```python
from build123d import *

# Parameters (mm, degrees)
BOSS_EXTRUDE1_DEPTH = 49.53
CUT_EXTRUDE1_DEPTH  = 44.45
SKETCH3_R           = 4.7625
CUT_EXTRUDE2_DEPTH  = 44.45


with BuildPart() as part:
    # Sketch1 → Boss-Extrude1 (new body)
    with BuildSketch(Plane(origin=(0, 0, 0), x_dir=(1, 0, 0), z_dir=(0, 1, 0))):
        Polygon((-12.7, -12.7), (-10.795, -12.7), (-10.795, -1.905), (10.795, -1.905), (10.795, -12.7), (12.7, -12.7), (12.7, 0), (-12.7, 0), align=None)
    extrude(amount=BOSS_EXTRUDE1_DEPTH)

    # Sketch2 → Cut-Extrude1 (cut)
    with BuildSketch(Plane(origin=(12.7, 0, 0), x_dir=(0, 0, -1), z_dir=(1, 0, 0))):
        with BuildLine():
            Line((-12.7, 0), (-8.821918242, 37.623946857))
            ThreePointArc((-8.821918242, 37.623946857), (-4.512325964, 46.11357553), (4.374429599, 49.53))
            Line((4.374429599, 49.53), (-12.7, 49.53))
            Line((-12.7, 49.53), (-12.7, 0))
        make_face()
    extrude(amount=-CUT_EXTRUDE1_DEPTH, mode=Mode.SUBTRACT)

    # Sketch3 → Cut-Extrude2 (cut)
    with BuildSketch(Plane(origin=(0, 0, 0), x_dir=(-1, 0, 0), z_dir=(0, 0, -1))):
        with Locations((0, 31.75)):
            Circle(SKETCH3_R)
        with BuildLine():
            Line((-12.115027858, 5.08), (-12.7, 5.08))
            Line((-12.7, 5.08), (-12.7, 0))
            Line((-12.7, 0), (12.7, 0))
            Line((12.7, 0), (12.7, 5.08))
            Line((12.7, 5.08), (12.115027858, 5.08))
            ThreePointArc((12.115027858, 5.08), (0, 13.97), (-12.115027858, 5.08))
        make_face()
    extrude(amount=-CUT_EXTRUDE2_DEPTH, mode=Mode.SUBTRACT)


solid = part.part
```
Read the model definition and answer for the solid it produces. Units are mm, in the model's axes. A direction names the side the tool comes from. Coordinates: 2 decimals unless noted, no trailing zeros. Write each loop counter-clockwise with the first axis right and the second up, starting at its lowest first coordinate (ties: lowest second). Pieces come first, ordered by that corner, then holes. Notation, with made-up numbers: (-21, 29) -> (26, 29) arc R13 ccw to (26, 50) -> close; hole circle Ø4 at (44.25, 5.5). An arc over 180 degrees is marked (long way). Write item = value, one per line.
(1) Section A-A on x = 0 is taken. Write down the section's boundary in (y, z) (1 decimal).
From the geometry:
outline = (14, 0) -> (27, 0) -> (27, 1.9) -> (14, 1.9) -> close; (36.5, 0) -> (48.8, 0) arc R13.3 ccw to (47.9, 1.9) -> (36.5, 1.9) -> close
(2) Given pin 1 Ø10 at (x, y) = (-1.5, 32) entering from +Z (3 decimals); pin 2 Ø3 at (x, y) = (7, 17) entering from -Z, each flat-ended and moving along its own axis, determine where each tip first touches the part or whether it passes through.
From the geometry:
pin_1 = 1.905
pin_2 = 0
(3) Section D-D on x = -3.5 is taken. Write down the section's boundary in (y, z) (3 decimals).
From the geometry:
outline = (13.478, 0) -> (28.52, 0) -> (28.52, 1.905) -> (13.478, 1.905) -> close; (34.98, 0) -> (48.788, 0) arc R13.266 ccw to (47.95, 1.905) -> (34.98, 1.905) -> close
(4) Section C-C on y = 39 is taken. Write down the section's boundary in (x, z) (3 decimals).
From the geometry:
outline = (-12.7, 0) -> (12.7, 0) -> (12.7, 8.607) -> (10.795, 8.607) -> (10.795, 1.905) -> (-10.795, 1.905) -> (-10.795, 8.607) -> (-12.7, 8.607) -> close
(5) Which of the six approach directions +Z, -Z, +X, -X, +Y, -Y give full straight-line access (tool end or side, diameter ignored) to faces 1 (the face through (11.761, 21.124, 10.523)), 2 (the face through (-10.795, 23, 6))?
From the geometry:
face_1 = +Z, +X, -X, +Y
face_2 = +Z, +Y, -Y
(6) Section B-B on y = 31.75 is taken. Write down the section's boundary in (x, z) (1 decimal).
From the geometry:
outline = (-12.7, 0) -> (-4.8, 0) -> (-4.8, 1.9) -> (-10.8, 1.9) -> (-10.8, 9.4) -> (-12.7, 9.4) -> close; (4.8, 0) -> (12.7, 0) -> (12.7, 9.4) -> (10.8, 9.4) -> (10.8, 1.9) -> (4.8, 1.9) -> close
(7) Straight lines are drawn through the part: L1, parallel to X at y = 39, z = 4.5 (3 decimals); L2, parallel to Z at x = 10, y = 25 (3 decimals); L3, parallel to X at y = 32, z = 0.75. For each, find the intervals that lie inside material, in ascending order. Write a range as from..to.
From the geometry:
L1 = -12.7..-10.795, 10.795..12.7
L2 = 0..1.905
L3 = -12.7..-4.76, 4.76..12.7
(8) For a pull along X with two mould halves and no side action, classify faces 3 (the face through (12.7, 22, 5)), 4 (the face through (-12.7, 22, 5)), 5 (the face through (-0.08, 13.97, 1.55)) as +X half, -X half, draft (parallel to the pull), parting line (faces both ways), or undercut.
From the geometry:
face_3 = +X half
face_4 = -X half
face_5 = undercut
